Study the drawing (mm; zero at the part's minimum x, y, z) and answer. A direction names the side the tool comes from. Give positions to 0.01 mm unless a question says otherwise; leave off trailing zeros. Write each loop counter-clockwise with the first axis right and the second up, starting at its lowest first coordinate (ties: lowest second). Pieces come first, ordered by that corner, then holes. Notation, with made-up numbers: M -1,88 L 34,88 A29 ccw 34,109 Z; hole C -12,-15 d4. An arc over 180 degrees is marked long. Use a Markdown table: item, result. Add a question column.
Item 1: Consider probe 1 along Y at (x, z) = (163.5, 13.5); probe 2 along Z at (x, y) = (149, 36) (1 decimal); probe 3 along Y at (x, z) = (149, 15.25). Determine where each line is inside the solid, lowest interval first. Write a range as [from, to].
Item 2: For the marked faces 1 and 2, determine the directions among +Z, -Z, +X, -X, +Y, -Y from which every point of the face is accessible in a straight line to the end or side of a thin tool.
Item 3: A cutting plane is placed at D-D on y = 71. Determine the outline of the cut face in (x, z).
Item 4: A cutting plane is placed at A-A on z = 12.7. Determine the outline of the cut face in (x, y) (1 decimal), then the cut area to 3 significant figures.
Item 5: A cutting plane is placed at C-C on x = 116. Determine the outline of the cut face in (y, z), then the cut area to 3 significant figures.
Item 6: Given P1, Ø4, axis at x = 144.5, z = 17.5, coming from the +Y side; P2, Ø2, axis at x = 110.5, z = 13, coming from the -Y side; P3, Ø4, axis at y = 59.5, z = 7, coming from the +X side, each flat-ended and moving along its own axis, determine where each tip first touches the part or whether it passes through.
Item 7: A cutting plane is placed at B-B on y = 49.5. Determine the outline of the cut face in (x, z) (1 decimal), then the cut area to 3 significant figures.
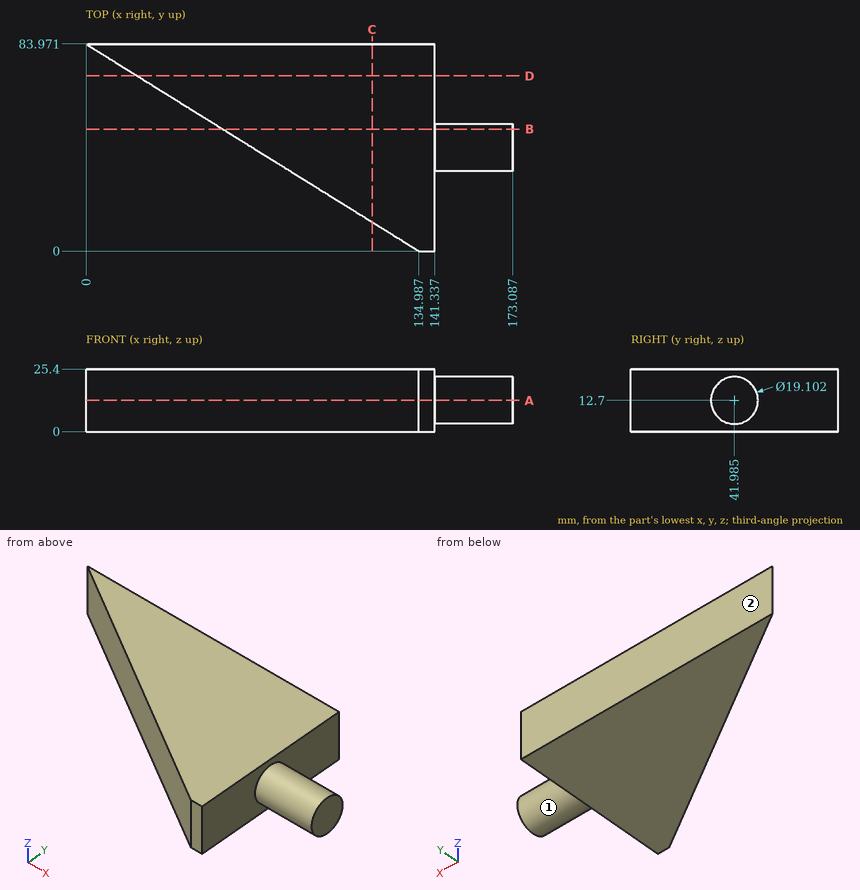
Filled in:
| question | item | result |
|---|---|---|
| 1 | probe 1 | [32.47, 51.5] |
| 1 | probe 2 | [5.3, 20.1] |
| 1 | probe 3 | [32.78, 51.19] |
| 2 | face 1 | +X |
| 2 | face 2 | +Z, -Z, +X, -X, +Y |
| 3 | outline | M 20.85,0 L 141.34,0 L 141.34,25.4 L 20.85,25.4 Z |
| 4 | outline | M 0,84 L 135,0 L 141.3,0 L 141.3,32.4 L 173.1,32.4 L 173.1,51.5 L 141.3,51.5 L 141.3,84 Z |
| 4 | area | 6,810 mm² |
| 5 | outline | M 11.81,0 L 83.97,0 L 83.97,25.4 L 11.81,25.4 Z |
| 5 | area | 1,830 mm² |
| 6 | P1 | y = 51.12 |
| 6 | P2 | y = 14.61 |
| 6 | P3 | x = 141.34 |
| 7 | outline | M 55.4,0 L 141.3,0 L 141.3,6.8 L 173.1,6.8 L 173.1,18.6 L 141.3,18.6 L 141.3,25.4 L 55.4,25.4 Z |
| 7 | area | 2,560 mm² |
